Check sheet for the modelled part. Datum: model origin and axes. Units: mm. A direction names the side the tool comes from. Round coordinates to 2 decimals unless told otherwise and drop trailing zeros. Loops run counter-clockwise (first coordinate to the right, second up) from the corner with the lowest first, then second, coordinate; pieces in that order, holes last. Notation, with made-up numbers: (28.5, 70) -> (72.5, 70) arc R28 cw to (72.5, 105) -> close; hole circle Ø9 at (80, 39). An arc over 180 degrees is marked (long way). Return JSON: item names as keys, results as strings.
Autodesk Inventor part; units mm, degrees
ref_plane "Work Plane1" through (1.525, 0, 0) normal (0, 0, 1) x (1, 0, 0)
ref_plane "YZ Plane" through (0, 0, 0) normal (1, 0, 0) x (0, 1, 0)
ref_plane "XZ Plane" through (0, 0, 0) normal (0, 1, 0) x (-1, 0, 0)
sketch "Sketch1" plane through (0, 0, 0) normal (0, 0, 1) x (1, 0, 0)
  line L0 (0, 7.1374) -> (0, 4.9276)
  line L1 (158.75, 4.7625) -> (190.5, 4.7625)
  line L2 (190.5, 4.7625) -> (190.5, 0)
  line L3 (190.5, 0) -> (-0.0001, 0)
  line L4 (-38.1001, 0) -> (228.6, 0)
  line L5 (-0.0001, 0) -> (-0.0001, 7.1374)
  line L6 (-0.0001, 7.1374) -> (0, 7.1374)
  line L7 (158.75, 4.7625) -> (154.7812, 4.9276)
  line L8 (154.7812, 4.9276) -> (0, 4.9276)
  line L9 (0, -1.4275) -> (0, 8.5649)
  dimension "d0" = 190.5
  dimension "d1" = 31.75
  dimension "d2" = 9.525
  dimension "d9" = 0.0001
  dimension "d10" = 14.2748
  dimension "d13" = 3.9689
  dimension "d14" = 9.8552
revolve "Body" add sketch "Sketch1" angle 360 about axis through (190.5, 0, 0) along (-1, 0, 0)
sketch "Sketch2" plane through (-0.0001, 0, 0) normal (-1, 0, 0) x (0, 0, 1)
  line L0 (0, 8.2416) -> (7.1374, 4.1208)
  line L1 (7.1374, 4.1208) -> (7.1374, -4.1208)
  line L2 (7.1374, -4.1208) -> (0, -8.2416)
  line L3 (0, -8.2416) -> (-7.1374, -4.1208)
  line L4 (-7.1374, -4.1208) -> (-7.1374, 4.1208)
  line L5 (-7.1374, 4.1208) -> (0, 8.2416)
  point P0 (0, 0)
  point P1 (0, 0)
  dimension "d11" = 14.2748
extrude "Head" add sketch "Sketch2" along normal blind 6.8072
sketch "Sketch4" plane through (0, 0, 0) normal (0, 0, 1) x (1, 0, 0)
  line L0 (-6.8073, 7.1374) -> (-6.8073, 8.2416)
  line L1 (-6.8073, 8.2416) -> (-6.1698, 8.2416)
  line L2 (-6.1698, 8.2416) -> (-6.8073, 7.1374)
  line L3 (-8.1687, 0) -> (1.3613, 0)
  line L4 (-0.0001, 8.2416) -> (-6.8073, 8.2416)
  line L5 (-6.8073, 4.1208) -> (-6.8073, 8.2416)
  dimension "d5" = 30
  dimension "d19" = 14.2748
revolve "Chamfer1" cut sketch "Sketch4" angle 360 about axis through (-10, 0, 0) along (1, 0, 0)
thread "Thread"
chamfer "Chamfer2" distance 0.9739 distance2 0.9447 1 edges at (190.5, -4.7625, 0) measured on face at (190.5, 0.2241, 1.3065)
ref_plane "Work Plane1" through (1.525, 0, 0) normal (0, 0, 1) x (1, 0, 0)
fillet "Fillet2" radius 0.762 1 edges at (0, -4.9276, 0)
equation "\"d63\" = R"
equation "\"d11\" = SW"
equation "\"d3\" = KOH - SD"
equation "\"d15\" = GEL"
equation "\"d6\" = -0.5 * SPD + 0.5 * GD"
equation "\"d0\" = NLG"
equation "\"d1\" = GEL"
equation "\"d2\" = GD"
equation "\"d10\" = SD2"
equation "\"d14\" = BDM"
equation "\"d5\" = ANG1"
equation "\"d19\" = SW0"
equation "\"NLG\" = 190.5"
equation "\"GD\" = NND"
equation "\"BDM\" = 9.8552"
equation "\"KOH\" = 6.8072"
equation "\"GEL\" = 31.75"
equation "\"SW\" = 14.2748"
equation "\"SW0\" = SW"
equation "\"SPD\" = GD1"
equation "\"SD2\" = SW"
equation "\"SD\" = 0"
equation "\"ANG1\" = 30deg"
equation "\"GAL\" = 3.96875"
equation "\"GUL\" = 0.238 * GAL"
equation "\"R\" = 0.762"
equation "\"d62\" = -NLG - SD + GUL"
equation "\"GD1\" = 7.5773"
equation "\"THREADDIA\" = 9.525"
equation "\"TOA\" = 30deg"
equation "\"NND\" = 9.525"
equation "\"E0\" = 1.155 * SW"
properties part number "am-1055" material "Steel, Mild"
Q1. Material ranges on line 1 (X direction, y = 2.5, z = -5.5); line 2 (Z direction, x = 66.5, y = -1.25); line 3 (Y direction, x = 105.5, z = 2.75), recorded low to high.
Results list:
{"line 1": "-6.81 to 0", "line 2": "-4.77 to 4.77", "line 3": "-4.09 to 4.09"}
Q2. Draft check along X on faces 3 (the flat face through (-3.36, -6.21, -3.52)), 4 (the flat face through (-6.807, 0, 0)), 5 (the flat face through (0, -6, 0)). Enter one of: released by +X, released by -X, zero draft, split by the parting line, or undercut.
Results list:
{"face 3": "zero draft", "face 4": "released by -X", "face 5": "released by +X"}
Q3. Tool access check on faces 1 (the flat face through (-3.36, 6.21, 3.52)), 2 (the cylindrical face through (76.693, -4.923, -0.217)). Record the directions out of +Z, -Z, +X, -X, +Y, -Y that give a thin tool (end or side, any length) a straight path to the whole face; none if there is none.
Results list:
{"face 1": "+Z, +X, -X, +Y", "face 2": "+X"}
Q4. Go/stop test with flat-tipped pins: pin 1 (1.5 mm diameter, centred on y = -0.5, z = -5, fed in from +X); pin 2 (1 mm diameter, centred on x = 97, y = -5, fed in from +Z); pin 3 (1 mm diameter, centred on x = 78, z = -5, fed in from -Y); pin 4 (1 mm diameter, centred on x = 154, y = -6.5, fed in from +Z). Record where each tip stops, or that it passes through.
Results list:
{"pin 1": "x = 190.03", "pin 2": "z = 2.01", "pin 3": "y = -2.01", "pin 4": "through"}
Q5. Section check A-A (x = 70.5). Record the boundary of the cut face in (y, z), then the cut area to 3 significant figures.
Results list:
{"outline": "circle Ø9.86 at (0, 0)", "area": "76.3 mm^2"}
